The listing builds one solid part. Answer for the finished solid, in the listing's coordinates (mm). Round coordinates to 2 decimals unless told otherwise and drop trailing zeros. Write each loop counter-clockwise with the first axis right and the second up, starting at its lowest first coordinate (ties: lowest second). Pieces come first, ordered by that corner, then holes. Notation, with made-up numbers: M 60,71 L 117,71 A17 ccw 117,97 Z; hole C 39,3 d6. An arc over 180 degrees is marked long. Write each question's results on one line, items separated by ' | '.
from build123d import *

# Parameters (mm, degrees)
SKETCH1_R           = 41.91
SKETCH1_R_2         = 2.5527
SKETCH1_R_3         = 12.7
BOSS_EXTRUDE1_DEPTH = 9.525


with BuildPart() as part:
    # Sketch1 → Boss-Extrude1 (new body)
    with BuildSketch(Plane.XY):
        with Locations(Location((0, 0, 0), (0, 0, 180))):
            Circle(SKETCH1_R)
        with Locations(Location((0, 23.8125, 0), (0, 0, 180))):
            Circle(SKETCH1_R_2, mode=Mode.SUBTRACT)
        with Locations(Location((20.622229928, 11.90625, 0), (0, 0, 180))):
            Circle(SKETCH1_R_2, mode=Mode.SUBTRACT)
        with Locations(Location((20.622229928, -11.90625, 0), (0, 0, 180))):
            Circle(SKETCH1_R_2, mode=Mode.SUBTRACT)
        with Locations(Location((0, -23.8125, 0), (0, 0, 180))):
            Circle(SKETCH1_R_2, mode=Mode.SUBTRACT)
        with Locations(Location((-20.622229928, -11.90625, 0), (0, 0, 180))):
            Circle(SKETCH1_R_2, mode=Mode.SUBTRACT)
        with Locations(Location((-20.622229928, 11.90625, 0), (0, 0, 180))):
            Circle(SKETCH1_R_2, mode=Mode.SUBTRACT)
        with Locations(Location((0, 0, 0), (0, 0, 180))):
            Circle(SKETCH1_R_3, mode=Mode.SUBTRACT)
    extrude(amount=BOSS_EXTRUDE1_DEPTH)


solid = part.part
1) Each of these flat-tipped pins is pushed along its axis until it touches: pin 1 (4 mm diameter, centred on y = -20.5, z = 4.5, fed in from -X); pin 2 (10 mm diameter, centred on x = -1, y = 30.5, fed in from -Z). Where does it stop, or does it pass through?
Return value:
pin 1: x = -37.61 | pin 2: z = 0
2) Section B-B (x = 0) is taken. Determine the outline of the cut face in (y, z) (3 decimals), then the cut area to 3 significant figures.
Return value:
outline: M -41.91,0 L -26.365,0 L -26.365,9.525 L -41.91,9.525 Z; M -21.26,0 L -12.7,0 L -12.7,9.525 L -21.26,9.525 Z; M 12.7,0 L 21.26,0 L 21.26,9.525 L 12.7,9.525 Z; M 26.365,0 L 41.91,0 L 41.91,9.525 L 26.365,9.525 Z | area: 459 mm²
3) Find the intervals of material crossed by line 1 (Y direction, x = 0, z = 5); line 2 (Y direction, x = -18.5, z = 3.25); line 3 (Y direction, x = -19, z = 7.25), in increasing order.
Return value:
line 1: -41.91 to -26.37, -21.26 to -12.7, 12.7 to 21.26, 26.37 to 41.91 | line 2: -37.61 to -13.32, -10.49 to 10.49, 13.32 to 37.61 | line 3: -37.36 to -13.88, -9.94 to 9.94, 13.88 to 37.36
4) The mould has two halves that part along X. Classify faces 1 (the face through (5.456, -41.553, 4.696)), 2 (the face through (-9, -10, 9.525)), 3 (the face through (-5.86, 11.267, 4.696)): +X half, -X half, draft (parallel to the pull), parting line (faces both ways), or undercut.
Return value:
face 1: parting line | face 2: draft | face 3: undercut
5) Section A-A (y = 0) is taken. Determine the outline of the cut face in (x, z) (3 decimals), then the cut area to 3 significant figures.
Return value:
outline: M -41.91,0 L -12.7,0 L -12.7,9.525 L -41.91,9.525 Z; M 12.7,0 L 41.91,0 L 41.91,9.525 L 12.7,9.525 Z | area: 556 mm²
6) Section C-C (x = -8.5) is taken. Determine the outline of the cut face in (y, z) (3 decimals), then the cut area to 3 significant figures.
Return value:
outline: M -41.039,0 L -9.436,0 L -9.436,9.525 L -41.039,9.525 Z; M 9.436,0 L 41.039,0 L 41.039,9.525 L 9.436,9.525 Z | area: 602 mm²
7) Section D-D (z = 4.5) is taken. Determine the outline of the cut face in (x, y).
Return value:
outline: C 0,0 d83.82; hole C -20.62,-11.91 d5.11; hole C -20.62,11.91 d5.11; hole C 0,0 d25.4; hole C 0,-23.81 d5.11; hole C 0,23.81 d5.11; hole C 20.62,-11.91 d5.11; hole C 20.62,11.91 d5.11
